Autodesk Inventor part; units mm, degrees
ref_plane "YZ Plane" through (0, 0, 0) normal (1, 0, 0) x (0, 1, 0)
ref_plane "XZ Plane" through (0, 0, 0) normal (0, 1, 0) x (-1, 0, 0)
ref_plane "XY Plane" through (0, 0, 0) normal (0, 0, 1) x (1, 0, 0)
sketch "Sketch1" plane through (0, 0, 0) normal (0, 1, 0) x (-1, 0, 0)
  line L0 (25.4, 12.7) -> (-25.4, 12.7)
  line L1 (-25.4, 12.7) -> (-25.4, -12.7)
  line L2 (-25.4, -12.7) -> (25.4, -12.7)
  line L3 (25.4, -12.7) -> (25.4, 12.7)
  line L4 (25.4, 12.7) -> (-25.4, -12.7) construction
  line L5 (-25.4, 12.7) -> (25.4, -12.7) construction
  line L6 (22.225, 9.525) -> (-22.225, 9.525)
  line L7 (-22.225, 9.525) -> (-22.225, -9.525)
  line L8 (-22.225, -9.525) -> (22.225, -9.525)
  line L9 (22.225, -9.525) -> (22.225, 9.525)
  line L10 (22.225, 9.525) -> (-22.225, -9.525) construction
  line L11 (-22.225, 9.525) -> (22.225, -9.525) construction
  point P0 (0, 0)
  dimension "d0" = 50.8
  dimension "d1" = 25.4
  dimension "d2" = 44.45
  dimension "d3" = 19.05
extrude "Extrusion1" add sketch "Sketch1" along normal blind 228.6
sketch "Sketch2" plane through (-25.4, 0, 12.7) normal (0, 0, 1) x (1, 0, 0)
  line L0 (50.8, 0) -> (50.8, 228.6)
  line L1 (0, 228.6) -> (50.8, 228.6)
  line L2 (0, 0) -> (0, 228.6)
  line L3 (25.4, 228.6) -> (25.4, 203.2)
  circle A0 centre (25.4, 203.2) radius 6.35
  line L4 (25.4, 203.2) -> (25.4, 25.4)
  line L5 (25.4, 203.2) -> (203.2, 203.2) construction
  line L6 (25.4, 25.4) -> (50.8, 25.4)
  line L7 (50.8, 25.4) -> (0, 25.4)
  line L8 (25.4, 25.4) -> (25.4, 19.05)
  line L9 (25.4, 25.4) -> (31.75, 25.4) construction
  line L10 (25.4, 19.05) -> (50.8, 19.05)
  line L11 (25.4, 19.05) -> (0, 19.05)
  line L12 (25.4, 19.05) -> (38.1, 19.05)
  line L13 (38.1, 19.05) -> (19.05, 19.05)
  circle A1 centre (38.1, 19.05) radius 2.54
  circle A2 centre (19.05, 19.05) radius 2.54
  point P0 (25.4, 0)
  dimension "d6" = 25.4
  dimension "d7" = 12.7
  dimension "d8" = 177.8
  dimension "d9" = 90
  dimension "d10" = 6.35
  dimension "d11" = 90
  dimension "d12" = 12.7
  dimension "d13" = 19.05
  dimension "d14" = 0
  dimension "d15" = 5.08
  dimension "d16" = 5.08
extrude "Extrusion2" cut sketch "Sketch2" against normal blind 228.6 contours A1 L10 | L10 A1 | L4 L3 A0 | A0 L3 L4 | A2 L11 | L11 A2
sketch "Sketch3" plane through (0, 0, 0) normal (0, -1, 0) x (1, 0, 0)
  line L0 (-22.225, -9.525) -> (-22.225, 9.525)
  line L1 (-22.225, 9.525) -> (22.225, 9.525)
  line L2 (22.225, 9.525) -> (22.225, -9.525)
  line L3 (22.225, -9.525) -> (-22.225, -9.525)
  line L4 (-25.4, 12.7) -> (25.4, 12.7)
  line L5 (-25.4, -12.7) -> (-25.4, 12.7)
  line L6 (25.4, -12.7) -> (-25.4, -12.7)
  line L7 (25.4, 12.7) -> (25.4, -12.7)
  point P0 (0, 0)
extrude "Extrusion3" cut sketch "Sketch3" against normal blind 6.35
sketch "Sketch4" plane through (-25.4, 228.6, 12.7) normal (0, 0, 1) x (1, 0, 0)
  line L0 (0, -222.25) -> (50.8, -222.25)
  line L1 (50.8, -222.25) -> (50.8, 0)
  line L2 (0, -222.25) -> (0, 0)
  line L3 (0, -209.55) -> (12.7, -222.25)
  line L4 (50.8, -209.55) -> (38.1, -222.25)
  point P0 (25.4, -228.6)
extrude "Extrusion4" cut sketch "Sketch4" against normal blind 635
sketch "Sketch5" plane through (-25.4, 228.6, 12.7) normal (0, 0, 1) x (1, 0, 0)
  line L0 (0, -209.55) -> (12.7, -222.25)
  line L1 (12.7, -222.25) -> (38.1, -222.25)
  line L2 (38.1, -222.25) -> (50.8, -209.55)
  line L3 (0, -209.55) -> (0, 0)
  line L4 (19.05, -222.25) -> (0, -203.2)
  point P0 (25.4, -228.6)
extrude "Extrusion5" cut sketch "Sketch5" against normal blind 635
sketch "Sketch6" plane through (-25.4, 228.6, 12.7) normal (0, 0, 1) x (1, 0, 0)
  line L0 (19.05, -222.25) -> (38.1, -222.25)
  line L1 (38.1, -222.25) -> (50.8, -209.55)
  line L2 (0, -203.2) -> (0, 0)
  line L3 (25.4, -222.25) -> (25.4, -158.75)
  line L4 (25.4, -222.25) -> (88.9, -222.25) construction
  circle A0 centre (25.4, -158.75) radius 9.525
  line L5 (25.4, -158.75) -> (43.3605, -140.7895)
  line L6 (25.4, -158.75) -> (50.8, -158.75) construction
  line L7 (43.3605, -140.7895) -> (7.4395, -176.7105)
  line L8 (7.4395, -176.7105) -> (43.3605, -176.7105)
  line L9 (43.3605, -176.7105) -> (43.3605, -140.7895)
  line L10 (43.3605, -140.7895) -> (7.4395, -140.7895)
  line L11 (7.4395, -140.7895) -> (7.4395, -176.7105)
  circle A1 centre (43.3605, -140.7895) radius 2.032
  circle A2 centre (7.4395, -140.7895) radius 2.032
  circle A3 centre (7.4395, -176.7105) radius 2.032
  circle A4 centre (43.3605, -176.7105) radius 2.032
  point P0 (25.4, -228.6)
  dimension "d25" = 63.5
  dimension "d26" = 90
  dimension "d27" = 19.05
  dimension "d28" = 25.4
  dimension "d29" = 45
  dimension "d30" = 50.8
  dimension "d31" = 4.064
  dimension "d32" = 4.064
  dimension "d33" = 4.064
  dimension "d34" = 4.064
extrude "Extrusion6" cut sketch "Sketch6" against normal blind 635 contours A0 L7 L3 | L3 L5 A0 | A3 L11 L8 | L8 L7 A3 | A4 L9 L8 | L8 L9 A4 | L7 A0 L5 | L11 A3 L7 | A2 L10 L11 | L11 L10 A2 | A1 L5 L9 | L9 L10 A1 | A1 L10 L5
sketch "Sketch7" plane through (-25.4, 228.6, 12.7) normal (0, 0, 1) x (1, 0, 0)
  circle A0 centre (25.4, -25.4) radius 6.35
  circle A1 centre (25.4, -25.4) radius 14.2875
  point P0 (25.4, -228.6)
  dimension "d37" = 28.575
extrude "Extrusion7" cut sketch "Sketch7" against normal blind 635
sketch "Sketch8" plane through (-25.4, 228.6, 12.7) normal (0, 0, 1) x (1, 0, 0)
  circle A0 centre (25.4, -158.75) radius 9.525
  circle A1 centre (25.4, -158.75) radius 14.2875
  point P0 (25.4, -228.6)
  dimension "d40" = 28.575
extrude "Extrusion8" cut sketch "Sketch8" against normal blind 25.4
properties part number "SuperStructure"
CAD build for the part. Positions are in the model's coordinates, mm. A direction names the side the tool comes from. Round coordinates to 2 decimals unless told otherwise and drop trailing zeros. Order: outer loops, then holes, each group sorted by start corner. A loop starts at its lowest first (then second) coordinate and runs counter-clockwise, first axis right, second up. Notation, with made-up numbers: (27.5, 40.5) - (54.5, 40.5) arc R11 cw to (54.5, 54.5) - close; hole circle Ø4 at (34, 49.25). An arc over 180 degrees is marked (long way). Answer in a Markdown table with one row per item. Add a question column.
(1) Band-saw the part on D-D on y = 192.5. List the corners of the cut face in (x, z) (3 decimals).
(2) 3-axis set-ups, long thin cutter, end or side, ignore diameter. For faces 1 (the face through (-6.9, 16.57, 11.13)), 2 (the face through (-22.225, 124, 0)): which of +Z, -Z, +X, -X, +Y, -Y reach the whole face in a straight line?
(3) Drop flat-ended pins along their axis: pin 1 Ø4.5 at (x, y) = (-17.96, 51.89) entering from +Z; pin 2 Ø8 at (x, z) = (-15.5, -1.5) entering from +Y. Give the stop position or say it passes through.
(4) Probe L1, parallel to Z at x = 1.5, y = 119 (3 decimals); L2, parallel to X at y = 144, z = -4 (3 decimals); L3, parallel to X at y = 21, z = 4 (3 decimals). List the from-to ranges inside material, lowest first. Write a range as [from, to].
(5) Mould opens along Z. For faces 3 (the face through (0, 116, -9.525)), 4 (the face through (23.37, 17.02, 0.18)), 5 (the face through (0, 116, -12.7)), 6 (the face through (0, 116, 9.525)) say: +Z half, -Z half, draft (parallel to the pull), parting line (faces both ways), or undercut.
(6) Band-saw the part on B-B on z = 0. List the corners of the cut face in (x, y) (3 decimals), and give its area (3 significant figures).
(7) Band-saw the part on A-A on x = 0. Count the separate pieces of the cut face and the enclosed holes in it, and give its area (3 significant figures).
(8) Band-saw the part on C-C on y = 166.5. List the corners of the cut face in (x, z) (3 decimals).
Data:
| question | item | result |
|---|---|---|
| 1 | outline | (-25.4, -12.7) - (-9.468, -12.7) - (-9.468, -9.525) - (-22.225, -9.525) - (-22.225, 9.525) - (-9.468, 9.525) - (-9.468, 12.7) - (-25.4, 12.7) - close; (9.468, -12.7) - (25.4, -12.7) - (25.4, 12.7) - (9.468, 12.7) - (9.468, 9.525) - (22.225, 9.525) - (22.225, -9.525) - (9.468, -9.525) - close |
| 2 | face 1 | +Z, -Z |
| 2 | face 2 | +Y, -Y |
| 3 | pin 1 | stops at z = 12.7 |
| 3 | pin 2 | passes through |
| 4 | L1 | z = [-12.7, -9.525], [9.525, 12.7] |
| 4 | L2 | x = [-25.4, -22.225], [22.225, 25.4] |
| 4 | L3 | x = [22.225, 25.4] |
| 5 | face 3 | undercut |
| 5 | face 4 | draft |
| 5 | face 5 | -Z half |
| 5 | face 6 | undercut |
| 6 | outline | (-25.4, 25.4) - (-22.225, 22.225) - (-22.225, 228.6) - (-25.4, 228.6) - close; (22.225, 15.875) - (25.4, 19.05) - (25.4, 228.6) - (22.225, 228.6) - close |
| 6 | area | 1,320 mm^2 |
| 7 | separate pieces | 6 |
| 7 | enclosed holes | 0 |
| 7 | area | 1,050 mm^2 |
| 8 | outline | (-25.4, -12.7) - (25.4, -12.7) - (25.4, 12.7) - (-25.4, 12.7) - close; hole (-22.225, -9.525) - (22.225, -9.525) - (22.225, 9.525) - (-22.225, 9.525) - close |
